Here's how the part is built. I have some questions about the finished solid (model axes, mm). Give positions to 0.01 mm unless a question says otherwise; leave off trailing zeros. Loops run counter-clockwise (first coordinate to the right, second up) from the corner with the lowest first, then second, coordinate; pieces in that order, holes last. Notation, with made-up numbers: (62.25, 77.5) - (75.25, 77.5) arc R29 ccw to (75.25, 114.5) - close; hole circle Ø9 at (7.5, -35). An arc over 180 degrees is marked (long way). Return JSON: item names as keys, results as strings. Group by question number.
(1) I need wall thicknesses on probe 1 along Y at (x, z) = (1, 3.3); probe 2 along X at (y, z) = (1.5, 3.35); probe 3 along Z at (x, y) = (-13.5, 7.5). Which ranges of each line are inside material? Lowest first, please. Write a range as [from, to].
(2) For P1, Ø1.5, axis at x = 23.5, y = 14, coming from the +Z side; P2, Ø0.5, axis at x = -11.5, z = 3.5, coming from the +Y side, each with a flat end and sliding along its axis, tell me the tip position at first contact or that it passes through.
(3) If we section it at A-A (y = 13.5): Please give me the cut outline in (x, z), then the cut area to 3 significant figures.
```python
from build123d import *

# Parameters (mm, degrees)
F0_W     = 60
F0_H     = 40
F1_DEPTH = 3
F2_R     = 0.644788
F3_DEPTH = 1


with BuildPart() as f1:
    # F0 (on Top) → F1 (new body)
    with BuildSketch(Plane.XY):
        Rectangle(F0_W, F0_H)
    extrude(amount=F1_DEPTH)

    # F2 (on face) → F3 (join)
    with BuildSketch(Plane.XY.offset(3)):
        with BuildLine():
            ThreePointArc((-1.83289, 4.985239), (-3.905066, 3.701445), (-5.582823, 1.933065))
            ThreePointArc((-5.582823, 1.933065), (-11.454748, 4.059319), (-17.675988, 4.603948))
            ThreePointArc((-17.675988, 4.603948), (-21.960088, 3.783559), (-24.130624, 0))
            ThreePointArc((-24.130624, 0), (-21.816485, -3.576152), (-17.972754, -5.411863))
            ThreePointArc((-17.972754, -5.411863), (-13.11323, -5.912843), (-8.253707, -5.411863))
            ThreePointArc((-8.253707, -5.411863), (-8.750343, -6.535326), (-9.292384, -7.637599))
            Line((-9.292384, -7.637599), (-13.007432, -7.637599))
            Line((-13.007432, -7.637599), (-9.992245, -8.657275))
            Line((-9.992245, -8.657275), (-9.992245, -9.32379))
            Line((-9.992245, -9.32379), (-12.975693, -9.958565))
            Line((-12.975693, -9.958565), (-9.40157, -10.466387))
            ThreePointArc((-9.40157, -10.466387), (0.779134, -14.859459), (10.959839, -10.466387))
            ThreePointArc((10.959839, -10.466387), (13.302708, -8.380835), (15.35197, -6.006159))
            ThreePointArc((15.35197, -6.006159), (14.817038, -2.212991), (12.276846, 0.65436))
            Line((12.276846, 0.65436), (16.732113, 4.702753))
            Line((16.732113, 4.702753), (11.768254, 1.590169))
            Line((11.768254, 1.590169), (14.189153, 6.818497))
            Line((14.189153, 6.818497), (10.58832, 1.590169))
            ThreePointArc((10.58832, 1.590169), (8.332541, 3.347539), (5.691082, 4.442793))
            ThreePointArc((5.691082, 4.442793), (6.116375, 10.969097), (3.898917, 17.121852))
            ThreePointArc((3.898917, 17.121852), (2.138019, 18.066027), (0.337851, 17.199064))
            ThreePointArc((0.337851, 17.199064), (-1.843688, 11.286972), (-1.83289, 4.985239))
        make_face()
        with BuildLine():
            ThreePointArc((-16.881408, 3.753243), (-10.934, 3.001613), (-5.359556, 0.796576))
            ThreePointArc((-5.359556, 0.796576), (-0.360554, 3.835426), (5.475548, 3.429784))
            ThreePointArc((5.475548, 3.429784), (8.143257, 2.076287), (10.519474, 0.259086))
            ThreePointArc((10.519474, 0.259086), (13.137989, -1.406759), (14.542523, -4.174239))
            ThreePointArc((14.542523, -4.174239), (14.542426, -5.421421), (13.926209, -6.505736))
            ThreePointArc((13.926209, -6.505736), (7.417681, -12.145032), (-1.009353, -13.919206))
            ThreePointArc((-1.009353, -13.919206), (-5.238705, -12.765816), (-8.291389, -9.619573))
            ThreePointArc((-8.291389, -9.619573), (-8.012131, -6.67233), (-6.334951, -4.232804))
            ThreePointArc((-6.334951, -4.232804), (-12.5061, -5.009925), (-18.710274, -4.568096))
            ThreePointArc((-18.710274, -4.568096), (-21.679234, -2.77657), (-23.069071, 0.400322))
            ThreePointArc((-23.069071, 0.400322), (-20.659117, 3.338847), (-16.881408, 3.753243))
        make_face(mode=Mode.SUBTRACT)
        with BuildLine():
            ThreePointArc((3.385171, 16.296154), (5.408767, 10.671196), (4.671817, 4.738912))
            ThreePointArc((4.671817, 4.738912), (3.965382, 5.075268), (3.362598, 5.574104))
            ThreePointArc((3.362598, 5.574104), (1.751569, 10.604004), (2.241873, 15.862798))
            Line((2.241873, 15.862798), (2.090248, 15.862798))
            ThreePointArc((2.090248, 15.862798), (1.321883, 10.754523), (2.324252, 5.686968))
            ThreePointArc((2.324252, 5.686968), (0.823876, 5.275564), (-0.700495, 4.96464))
            ThreePointArc((-0.700495, 4.96464), (-1.037753, 10.93409), (0.90217, 16.589599))
            ThreePointArc((0.90217, 16.589599), (2.215281, 17.048816), (3.385171, 16.296154))
        make_face(mode=Mode.SUBTRACT)
        with BuildLine():
            ThreePointArc((3.027315, -2.605882), (2.311567, -2.050264), (1.427228, -1.8529))
            ThreePointArc((1.427228, -1.8529), (-0.272035, -2.308318), (-0.800345, -3.98635))
            ThreePointArc((-0.800345, -3.98635), (0.170039, -5.458062), (1.919497, -5.24132))
            ThreePointArc((1.919497, -5.24132), (3.083669, -4.180128), (3.027315, -2.605882))
        make_face()
        with Locations((1.427228, -3.139245)):
            Circle(F2_R, mode=Mode.SUBTRACT)
        with BuildLine():
            ThreePointArc((8.07857, 0.280549), (7.398587, 0.631767), (6.635354, 0.688415))
            ThreePointArc((6.635354, 0.688415), (5.214115, -0.287698), (5.12939, -2.009772))
            ThreePointArc((5.12939, -2.009772), (6.714717, -2.684062), (8.392313, -2.29214))
            ThreePointArc((8.392313, -2.29214), (9.02358, -0.909681), (8.07857, 0.280549))
        make_face()
        with Locations((6.480221, -0.763344)):
            Circle(F2_R, mode=Mode.SUBTRACT)
        with BuildLine():
            ThreePointArc((7.168717, -4.017724), (6.306207, -4.355034), (5.380385, -4.331466))
            ThreePointArc((5.380385, -4.331466), (4.763195, -5.429565), (5.380385, -6.527665))
            Line((5.380385, -6.527665), (6.070618, -6.49629))
            ThreePointArc((6.070618, -6.49629), (7.335615, -6.766785), (8.235442, -5.837431))
            ThreePointArc((8.235442, -5.837431), (8.175536, -4.650034), (7.168717, -4.017724))
        make_face()
        with BuildLine():
            ThreePointArc((5.363596, -9.458974), (3.596654, -10.093438), (2.020633, -9.073249))
            ThreePointArc((2.020633, -9.073249), (1.352594, -9.275514), (1.334897, -9.973277))
            ThreePointArc((1.334897, -9.973277), (3.309765, -11.368484), (5.577887, -10.530437))
            ThreePointArc((5.577887, -10.530437), (5.827257, -9.923403), (5.363596, -9.458974))
        make_face()
        with BuildLine():
            ThreePointArc((-21.25046, 0.778031), (-17.402552, 2.364946), (-13.349544, 1.417411))
            ThreePointArc((-13.349544, 1.417411), (-11.052781, -0.571642), (-8.097489, -1.277121))
            ThreePointArc((-8.097489, -1.277121), (-6.992115, -1.425307), (-5.950998, -1.825162))
            ThreePointArc((-5.950998, -1.825162), (-5.435611, -1.813036), (-5.174607, -1.368461))
            ThreePointArc((-5.174607, -1.368461), (-6.777898, -0.155153), (-8.78254, 0))
            ThreePointArc((-8.78254, 0), (-10.277191, 0.101942), (-11.614082, 0.778031))
            ThreePointArc((-11.614082, 0.778031), (-13.17973, 2.239961), (-15.176346, 3.015862))
            ThreePointArc((-15.176346, 3.015862), (-18.581793, 2.896863), (-21.25046, 0.778031))
        make_face()
    extrude(amount=F3_DEPTH)


solid = f1.part
```
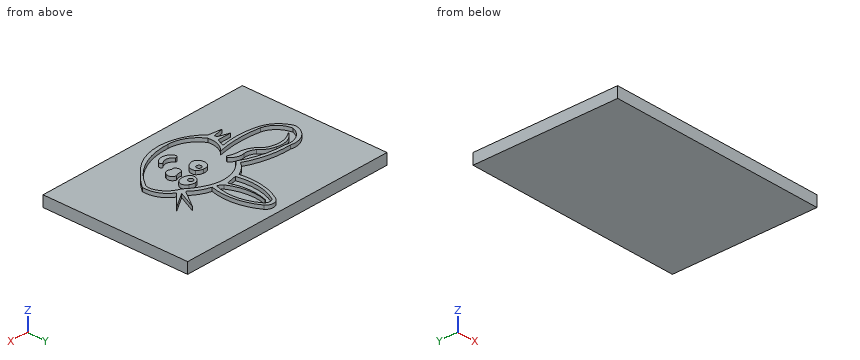
Values:
{
 "1": {"probe 1": "[-14.86, -13.89], [-5.61, -3.62], [-2.66, -1.8], [4.06, 5.32], [16.68, 17.78]", "probe 2": "[-23.77, -22.58], [-20.68, -20.21], [-13.49, -12.24], [-6.75, -4.68], [9, 13.21]", "probe 3": "[0, 3]"},
 "2": {"P1": "z = 3", "P2": "y = 4.12"},
 "3": {"outline": "(-30, 0) - (30, 0) - (30, 3) - (5.55, 3) - (5.55, 4) - (4.76, 4) - (4.76, 3) - (1.76, 3) - (1.76, 4) - (1.51, 4) - (1.51, 3) - (-0.46, 3) - (-0.46, 4) - (-1.3, 4) - (-1.3, 3) - (-30, 3) - close", "area": "182 mm2"}
}
